Build history of the part. All positions in model axes, mm. A direction names the side the tool comes from. Coordinates: 2 decimals unless noted, no trailing zeros. Write each loop counter-clockwise with the first axis right and the second up, starting at its lowest first coordinate (ties: lowest second). Pieces come first, ordered by that corner, then holes. Notation, with made-up numbers: (69, -28.5) -> (111, -28.5) arc R12 cw to (111, -11.5) -> close; hole circle Ø6 at (48, 65). An arc over 180 degrees is marked (long way). Write each question's results on one line, items separated by ' | '. Start each with the question number.
Q1. Saw through at C-C on x = 37.5. Give the cut face in (y, z), and give its area (3 significant figures).
Q2. Saw through at A-A on y = 0. Give the cut face in (x, z), and give its area (3 significant figures).
Q3. Saw through at D-D on y = 4.25. Give the cut face in (x, z), and give its area (3 significant figures).
Q4. Two-plate mould, pull along Y, no slides. Class faces 5 (the face through (25, -12.5, -1)), 6 (the face through (3, 2, 3)), 7 (the face through (0, -10, -1)): released by +Y, released by -Y, zero draft, split by the parting line, or undercut.
Q5. Drill centre lines: line 1 (Y direction, x = 0.7, z = 0); line 2 (Y direction, x = -0.3, z = 0); line 3 (X direction, y = -4.25, z = 0.5). Where is each one in solid material? Low to high.
Q6. Saw through at B-B on z = 0. Give the cut face in (x, y), and give its area (3 significant figures).
Q7. Drop flat-ended pins along their axis: pin 1 Ø10 at (x, z) = (19, -8) entering from +Y; pin 2 Ø2.5 at (y, z) = (9.5, 0.5) entering from -X; pin 3 Ø1.5 at (x, y) = (15, 0) entering from -Z. Give the stop position or say it passes through.
Q8. Tool access for faces 1 (the face through (26.171, 10.656, 3.356)), 2 (the face through (26, 0, -12.5)), 3 (the face through (-0.5, 0, -4)), 4 (the face through (0, 10, -1)): list every direction of +Z, -Z, +X, -X, +Y, -Y with a clear straight run to the whole face (end or side of a thin tool).
from build123d import *

# Parameters (mm, degrees)
F0_R     = 11.171963
F0_R_2   = 3.25
F1_DEPTH = 3
F0_W     = 25
F0_H     = 25
F2_DEPTH = 50
F3_DEPTH = 3
F4_W     = 15.2
F4_H     = 27.411
F4_R     = 3.25
F5_DEPTH = 0.5


with BuildPart() as f1:
    # F0 (on Right) → F1 (new body)
    with BuildSketch(Plane.YZ):
        Circle(F0_R)
        Circle(F0_R_2, mode=Mode.SUBTRACT)
    extrude(amount=F1_DEPTH)

    # F0 (on Right) → F2 (join)
    with BuildSketch(Plane.YZ):
        Rectangle(F0_W, F0_H)
        Circle(F0_R, mode=Mode.SUBTRACT)
    extrude(amount=F2_DEPTH)

    # F0 (on Right) → F3 (join)
    with BuildSketch(Plane.YZ):
        Polygon((12.52148, -14.911), (12.5, -12.5), (-12.5, -12.5), (-12.5, -14.911), align=None)
    extrude(amount=F3_DEPTH)

    # F4 (on face) → F5 (join)
    with BuildSketch(Plane(origin=(0, 0, 0), x_dir=(0, -1, 0), z_dir=(-1, 0, 0))):
        with Locations((0.1, -1.2055)):
            Rectangle(F4_W, F4_H)
        Circle(F4_R, mode=Mode.SUBTRACT)
    extrude(amount=F5_DEPTH)


solid = f1.part
Returned:
1) outline: (-12.5, -12.5) -> (12.5, -12.5) -> (12.5, 12.5) -> (-12.5, 12.5) -> close; hole circle Ø22.34 at (0, 0) | area: 233 mm2
2) outline: (-0.5, -14.91) -> (3, -14.91) -> (3, -12.5) -> (50, -12.5) -> (50, -11.17) -> (3, -11.17) -> (3, -3.25) -> (-0.5, -3.25) -> close; (-0.5, 3.25) -> (3, 3.25) -> (3, 11.17) -> (50, 11.17) -> (50, 12.5) -> (-0.5, 12.5) -> close | area: 198 mm2
3) outline: (-0.5, -14.91) -> (3, -14.91) -> (3, -12.5) -> (50, -12.5) -> (50, -10.33) -> (3, -10.33) -> (3, 10.33) -> (50, 10.33) -> (50, 12.5) -> (-0.5, 12.5) -> close | area: 300 mm2
4) face 5: released by -Y | face 6: undercut | face 7: zero draft
5) line 1: y = -12.5 to -3.25, 3.25 to 12.5 | line 2: y = -7.7 to -3.25, 3.25 to 7.5 | line 3: x = -0.5 to 3
6) outline: (-0.5, -7.7) -> (0, -7.7) -> (0, -12.5) -> (50, -12.5) -> (50, -11.17) -> (3, -11.17) -> (3, -3.25) -> (-0.5, -3.25) -> close; (-0.5, 3.25) -> (3, 3.25) -> (3, 11.17) -> (50, 11.17) -> (50, 12.5) -> (0, 12.5) -> (0, 7.5) -> (-0.5, 7.5) -> close | area: 185 mm2
7) pin 1: stops at y = 12.5 | pin 2: stops at x = 0 | pin 3: stops at z = -12.5
8) face 1: +X | face 2: -Z, +X, +Y, -Y | face 3: +Z, -Z, -X, +Y, -Y | face 4: +Z, -Z, -X, +Y
